Study the drawing (mm; zero at the part's minimum x, y, z) and answer. A direction names the side the tool comes from. Give positions to 0.01 mm unless a question says otherwise; leave off trailing zeros. Order: outer loops, then holes, each group sorted by start corner. A loop starts at its lowest first (then second) coordinate and runs counter-clockwise, first axis right, second up.
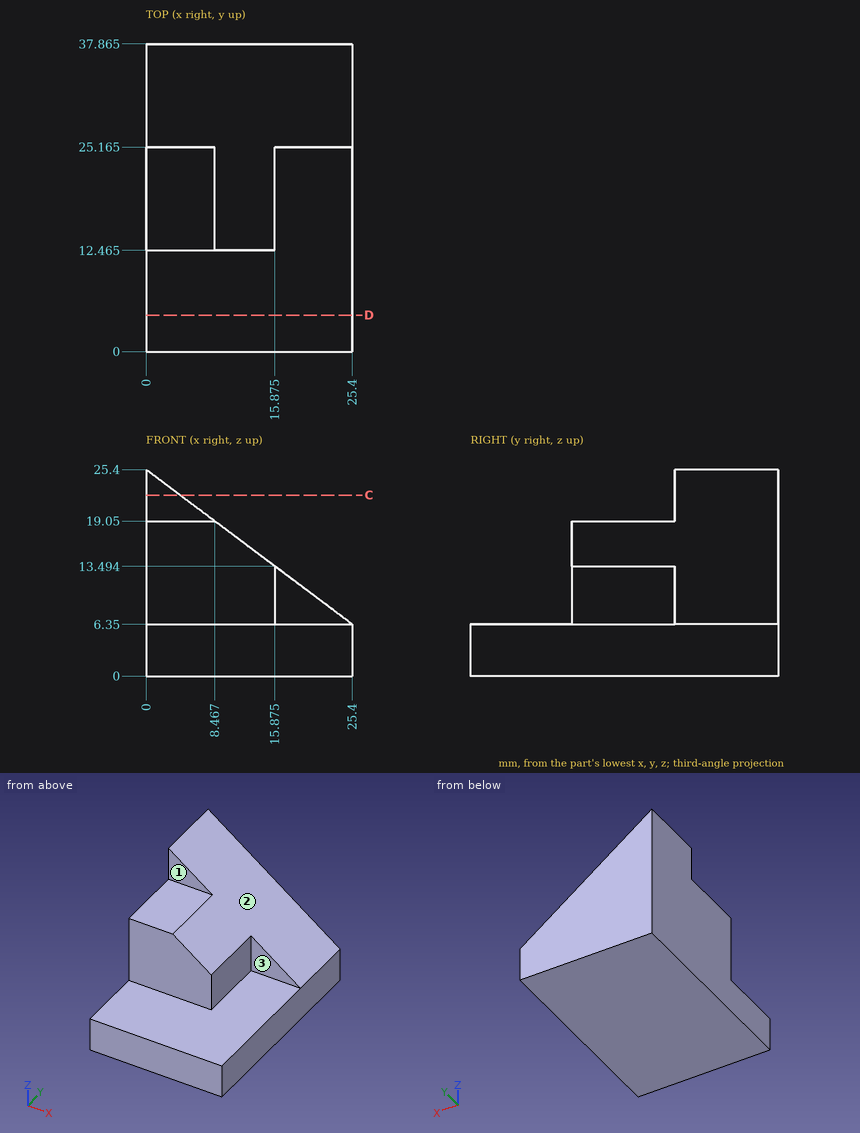
1) A tool of negligible diameter and unlimited length cuts with its end or side. For the marked faces 1, 2 and 3, from which of +Z, -Z, +X, -X, +Y, -Y can it reach the whole face along a straight path? Write none if from no direction.
Geometry says:
face 1: +Z, +X, -X, -Y
face 2: +Z, +X, +Y, -Y
face 3: +Z, +X, -Y
2) Find section D-D (y = 4.5). Write down the section's boundary in (x, z), then the cut area to 3 significant figures.
Geometry says:
outline: (0, 0) - (25.4, 0) - (25.4, 6.35) - (0, 6.35) - close
area: 161 mm2
3) Straight lines are drawn through the part: probe 1 along Z at (x, y) = (2.75, 2); probe 2 along X at (y, z) = (19.5, 13) (1 decimal); probe 3 along Y at (x, z) = (16.25, 11.25) (1 decimal). For each, find the intervals that lie inside material, in ascending order.
Geometry says:
probe 1: z = 0 to 6.35
probe 2: x = 0 to 15.9
probe 3: y = 25.2 to 37.9
4) Given P1, Ø4, axis at y = 27, z = 19, coming from the +X side; P2, Ø2, axis at x = 14, z = 11, coming from the -Y side (1 decimal); P3, Ø4, axis at x = 3, y = 20.5, coming from the +Z side; P4, Ø6.5, axis at x = 8.5, z = 9.5, coming from the -Y side, each flat-ended and moving along its own axis, determine where each tip first touches the part or whether it passes through.
Geometry says:
P1: stops at x = 11.2
P2: stops at y = 12.5
P3: stops at z = 19.05
P4: stops at y = 0
5) Find section C-C (z = 22.25). Write down the section's boundary in (x, y) (1 decimal).
Geometry says:
outline: (0, 25.2) - (4.2, 25.2) - (4.2, 37.9) - (0, 37.9) - close
